Design review of the part shown in the three views and the two pictorial views. Dimensions are in mm from the part's minimum x, y and z. A direction names the side the tool comes from. Give positions to 0.01 mm unless a question says otherwise; leave off trailing zeros. Loops run counter-clockwise (first coordinate to the right, second up) from the corner with the lowest first, then second, coordinate; pieces in that order, holes last. Notation, with made-up numbers: (-17, 79.5) -> (-6, 79.5) arc R22 ccw to (-6, 97.5) -> close; hole circle Ø3 at (17, -16). An arc over 180 degrees is marked (long way). Answer as CSV lines item,"result". Start each with the question number.
Item 1: Add section A-A on x = 36.2. State the section outline as (y, z) points, plus the area to 3 significant figures.
Item 2: Clearance check with flat-ended pins moving along their axes: P1, Ø2.5, axis at y = 60.5, z = 3.5, coming from the -X side; P2, Ø1.6, axis at x = 66.5, z = 3, coming from the +Y side; P3, Ø3, axis at y = 56.5, z = 0.5, coming from the +X side. State where each tip first meets the part, or that it passes through.
Item 3: The part is to be moulded in two halves that separate along Y. For the marked faces 1, 2 and 3, say which applies: +Y half, -Y half, draft (parallel to the pull), parting line (faces both ways), or undercut.
Item 4: Add section B-B on z = 4.05. State the section outline as (x, y) points.
Item 5: For L1, parallel to Y at x = 36.2, z = 1.15; L2, parallel to Y at x = 44, z = 0.8; L3, parallel to Y at x = 40.5, z = 2.5 (1 decimal), list the stretches that pass through material, from the lowest coordinate up. Write a range as from..to.
Item 6: Add section D-D on x = 63.5. State the section outline as (y, z) points, plus the area to 3 significant figures.
Item 7: Machinability: for the marked faces 4 and 5, which of the approach directions +Z, -Z, +X, -X, +Y, -Y give a long, thin tool a straight path to every point of the face, cutting with its end or side? Answer none if there is none.
Item 8: Add section C-C on y = 64.5. State the section outline as (x, z) points.
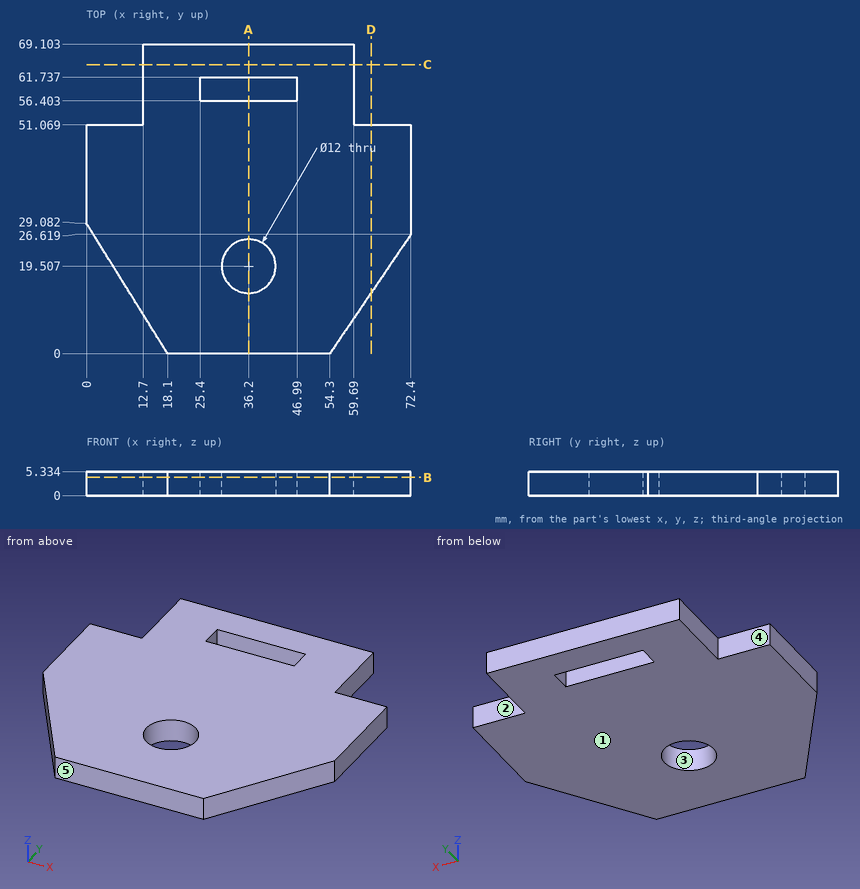
Computed values:
1,outline,"(0, 0) -> (13.51, 0) -> (13.51, 5.33) -> (0, 5.33) -> close; (25.51, 0) -> (56.4, 0) -> (56.4, 5.33) -> (25.51, 5.33) -> close; (61.74, 0) -> (69.1, 0) -> (69.1, 5.33) -> (61.74, 5.33) -> close"
1,area,"276 mm²"
2,P1,"x = 12.7"
2,P2,"y = 51.07"
2,P3,"x = 59.69"
3,face 1,"draft"
3,face 2,"+Y half"
3,face 3,"undercut"
4,outline,"(0, 29.08) -> (18.1, 0) -> (54.3, 0) -> (72.4, 26.62) -> (72.4, 51.07) -> (59.69, 51.07) -> (59.69, 69.1) -> (12.7, 69.1) -> (12.7, 51.07) -> (0, 51.07) -> close; hole (25.4, 56.4) -> (46.99, 56.4) -> (46.99, 61.74) -> (25.4, 61.74) -> close; hole circle Ø12 at (36.2, 19.51)"
5,L1,"0..13.51, 25.51..56.4, 61.74..69.1"
5,L2,"0..56.4, 61.74..69.1"
5,L3,"0..15.3, 23.7..56.4, 61.7..69.1"
6,outline,"(13.53, 0) -> (51.07, 0) -> (51.07, 5.33) -> (13.53, 5.33) -> close"
6,area,"200 mm²"
7,face 4,"+Z, -Z, -X, +Y"
7,face 5,"+Z, -Z, +X, -X, -Y"
8,outline,"(12.7, 0) -> (59.69, 0) -> (59.69, 5.33) -> (12.7, 5.33) -> close"
